Here's how the part is built. I have some questions about the finished solid (model axes, mm). A direction names the side the tool comes from. Round coordinates to 2 decimals unless told otherwise and drop trailing zeros. Write each loop counter-clockwise with the first axis right and the second up, starting at its lowest first coordinate (ties: lowest second). Pieces come first, ordered by that corner, then holes. Notation, with made-up numbers: (70, 10) -> (77, 10) arc R15 cw to (77, 29) -> close; hole circle Ø5 at (-21.5, 76). An arc over 180 degrees is marked (long way). Answer as CSV lines item,"result".
```python
from build123d import *

# Parameters (mm, degrees)
SKETCH1_R           = 55.88
BOSS_EXTRUDE1_DEPTH = 444.5
SKETCH4_R           = 12.7
BOSS_EXTRUDE3_DEPTH = 76.2


with BuildPart() as part:
    # Sketch1 → Boss-Extrude1 (new body)
    with BuildSketch(Plane.XY):
        Circle(SKETCH1_R)
    extrude(amount=BOSS_EXTRUDE1_DEPTH)

    # Sketch3 → Revolve1 (revolve)
    with BuildSketch(Plane(origin=(0, 0, 0), x_dir=(0, 0, -1), z_dir=(1, 0, 0)), mode=Mode.PRIVATE) as revolve1_sk:
        with BuildLine():
            Line((25.4, -12.7), (25.4, 0))
            Line((25.4, 0), (0, 0))
            Line((0, 0), (0, -55.88))
            ThreePointArc((0, -55.88), (19.362446334, -38.209086079), (25.4, -12.7))
        make_face()
    revolve(revolve1_sk.sketch.rotate(Axis((0, 0, 0), (0, 0, -1)), 270), axis=Axis((0, 0, 0), (0, 0, -1)))

    # Sketch4 → Boss-Extrude3 (add)
    with BuildSketch(Plane(origin=(0, 0, -25.4), x_dir=(-1, 0, 0), z_dir=(0, 0, -1))):
        with Locations(Location((0, 0, 0), (0, 0, 180))):
            Circle(SKETCH4_R)
    extrude(amount=BOSS_EXTRUDE3_DEPTH)


solid = part.part
```
1. If I drill on line 1 (Y direction, x = 0, z = 104); line 2 (X direction, y = 2.5, z = -18); line 3 (Z direction, x = -40, y = -37.5), over which ranges is the centre line in solid material (lowest first)?
Numbers:
line 1,"y = -55.88 to 55.88"
line 2,"x = -40.3 to 40.3"
line 3,"z = -2.09 to 444.5"
2. For pin 1 Ø8 at (x, y) = (-31, 36.5) entering from -Z; pin 2 Ø8 at (y, z) = (27, 40.5) entering from -X; pin 3 Ø3 at (x, z) = (-23.5, 2.5) entering from -Y, each with a flat end and sliding along its axis, tell me the tip position at first contact or that it passes through.
Numbers:
pin 1,"stops at z = -15.4"
pin 2,"stops at x = -50.93"
pin 3,"stops at y = -51.37"
3. Suppose I cut it at A-A on z = -36. Please give me the cut outline in (x, y).
Numbers:
outline,"circle Ø25.4 at (0, 0)"
4. On a 3-axis mill with a long thin cutter (end or side, diameter ignored), from which of +Z, -Z, +X, -X, +Y, -Y can I reach the whole of each face in a straight line? I mean faces 1 (the face through (5.86, 11.267, -62.967)), 2 (the face through (-7.3, 55.4, 219.1)). Say none if no direction works.
Numbers:
face 1,"-Z"
face 2,"+Z, -Z"
5. Suppose I cut it at B-B on z = 203.5. Please give me the cut outline in (x, y).
Numbers:
outline,"circle Ø111.76 at (0, 0)"
